Build history of the part. All positions in model axes, mm. A direction names the side the tool comes from. Round coordinates to 2 decimals unless told otherwise and drop trailing zeros. Order: outer loops, then holes, each group sorted by start corner. A loop starts at its lowest first (then second) coordinate and runs counter-clockwise, first axis right, second up. Notation, with made-up numbers: (-11.5, 34.25) -> (14.5, 34.25) arc R31 ccw to (14.5, 69.25) -> close; hole circle Ø11 at (-26, -18). An arc over 180 degrees is marked (long way). Write item = value, one per line.
from build123d import *

# Parameters (mm, degrees)
F1_DEPTH = 1000
F4_D     = 0.5


with BuildPart() as f1:
    # F0 (on Front) → F1 (new body)
    with BuildSketch(Plane.XZ):
        Polygon((400, 500), (-600, 500), (-600, -500), (600, -500), (600, -400), (400, -400), align=None)
    extrude(amount=F1_DEPTH)

    # F4 (through all)
    with Locations(Plane.YZ.offset(400)):
        with Locations((-500, -300)):
            Hole(F4_D / 2)


solid = f1.part
Q1. Flat gauge pin, fed straight in: pin 1 (5 mm diameter, centred on y = -420, z = 391.5, fed in from +X). Where does the tip first touch, or does it go through?
Check values:
pin_1 = 400
Q2. Cut at B-B, the plane z = 188. List the corners of the cut face in (x, y), and give its area (3 significant figures).
Check values:
outline = (-600, -1000) -> (400, -1000) -> (400, 0) -> (-600, 0) -> close
area = 1,000,000 mm²
Q3. Which spindle directions (+Z, -Z, +X, -X, +Y, -Y) get a long thin tool onto all of the face, cutting with end or side? Do faces 1 (the face through (600, -493, -451)), 2 (the face through (400, -493, 44)). Say none if no direction does.
Check values:
face_1 = +Z, -Z, +X, +Y, -Y
face_2 = +Z, +X, +Y, -Y
Q4. Probe probe 1 along Z at (x, y) = (-226, -500); probe 2 along Y at (x, z) = (-55, -300); probe 3 along X at (y, z) = (-490.5, 158). List the from-to ranges inside material, lowest first.
Check values:
probe_1 = -500 to -300.25, -299.75 to 500
probe_2 = -1000 to -500.25, -499.75 to 0
probe_3 = -600 to 400
Q5. Cut at A-A, the plane y = -95.5. List the corners of the cut face in (x, z), and give its area (3 significant figures).
Check values:
outline = (-600, -500) -> (600, -500) -> (600, -400) -> (400, -400) -> (400, 500) -> (-600, 500) -> close
area = 1,020,000 mm²
